Solid Edge part; units mm, degrees
sketch "Sketch1" plane through (0, 0, 0) normal (0, 0, 1) x (1, 0, 0)
  circle A0 centre (0, 41.891) radius 2.5
  line L0 (-5, 46.891) -> (5, 46.891)
  line L1 (5, 46.891) -> (5, 36.891)
  line L2 (5, 36.891) -> (-5, 36.891)
  line L3 (-5, 36.891) -> (-5, 46.891)
  circle A1 centre (0, -41.891) radius 2.5
  line L4 (-5, -46.891) -> (5, -46.891)
  line L5 (5, -46.891) -> (5, -36.891)
  line L6 (5, -36.891) -> (-5, -36.891)
  line L7 (-5, -36.891) -> (-5, -46.891)
  line L8 (-26, 36.891) -> (26, 36.891)
  line L9 (26, 36.891) -> (26, -36.891)
  line L10 (26, -36.891) -> (-26, -36.891)
  line L11 (-26, -36.891) -> (-26, 36.891)
  circle A2 centre (0, 15.851) radius 5
  dimension "D1" = 26
  dimension "D2" = 26
  dimension "D3" = 5
  dimension "D4" = 5
  dimension "D5" = 5
  dimension "D6" = 5
extrude "Protrusion1" add sketch "Sketch1" against normal blind 3
fillet "v_10" radius 10 4 edges at (26, -36.891, -1.5) (26, 36.891, -1.5) (-26, 36.891, -1.5) (-26, -36.891, -1.5)
fillet "v_5" radius 5 8 edges at (5, -46.891, -1.5) (-5, -46.891, -1.5) (5, -36.891, -1.5) (-5, -36.891, -1.5) (5, 46.891, -1.5) (5, 36.891, -1.5) (-5, 46.891, -1.5) (-5, 36.891, -1.5)
properties material "ABS Plastic, high impact"
The model under review builds one solid part; all positions refer to its coordinate system, in mm. A direction names the side the tool comes from. Give positions to 0.01 mm unless a question says otherwise; leave off trailing zeros. Write each loop counter-clockwise with the first axis right and the second up, starting at its lowest first coordinate (ties: lowest second). Pieces come first, ordered by that corner, then holes. Notation, with made-up numbers: M 29.25,-33.5 L 37.25,-33.5 A11 ccw 37.25,-17.5 Z; hole C 51,-17.5 d6. An arc over 180 degrees is marked long. Answer in a Markdown table with one row per item.
Item 1: Add section A-A on z = -0.8. State how many separate pieces and enclosed holes the cut face has, plus the area to 3 significant figures.
Check sheet entries:
| item | result |
|---|---|
| separate pieces | 1 |
| enclosed holes | 3 |
| area | 3,830 mm2 |
Item 2: Add section C-C on x = 7.5. Give the boundary of the cut face in (y, z), plus the area to 3 significant figures.
Check sheet entries:
| item | result |
|---|---|
| outline | M -37.56,-3 L 37.56,-3 L 37.56,0 L -37.56,0 Z |
| area | 225 mm2 |
Item 3: For line 1 along Y through (x, z) = (0, -2); line 2 along Y through (x, z) = (2, -1.1); line 3 along X through (y, z) = (18, -0.2), list the stretches that pass through material, from the lowest coordinate up.
Check sheet entries:
| item | result |
|---|---|
| line 1 | -46.89 to -44.39, -39.39 to 10.85, 20.85 to 39.39, 44.39 to 46.89 |
| line 2 | -46.47 to -43.39, -40.39 to 11.27, 20.43 to 40.39, 43.39 to 46.47 |
| line 3 | -26 to -4.51, 4.51 to 26 |
Item 4: Tool access review of faces 4 (the face through (0, 1, -3)), 5 (the face through (-13, -36.891, -1)), 6 (the face through (-13, 36.891, -1)), 7 (the face through (13, -36.891, -1)): name each direction out of +Z, -Z, +X, -X, +Y, -Y from which nothing blocks a thin tool from reaching the whole face with its end or side.
Check sheet entries:
| item | result |
|---|---|
| face 4 | -Z, +X, -X, +Y, -Y |
| face 5 | +Z, -Z, -X, -Y |
| face 6 | +Z, -Z, -X, +Y |
| face 7 | +Z, -Z, +X, -Y |
Item 5: Draft analysis for pull direction X (two halves, no side actions). For faces 1 (the face through (-0.54, -44.33, -1.48)), 2 (the face through (0, 1, 0)), 3 (the face through (3.497, 45.465, -1.521)), state which applies: +X half, -X half, draft (parallel to the pull), parting line (faces both ways), or undercut.
Check sheet entries:
| item | result |
|---|---|
| face 1 | undercut |
| face 2 | draft |
| face 3 | +X half |
Item 6: Add section B-B on x = -6. Give the boundary of the cut face in (y, z), plus the area to 3 significant figures.
Check sheet entries:
| item | result |
|---|---|
| outline | M -38.89,-3 L 38.89,-3 L 38.89,0 L -38.89,0 Z |
| area | 233 mm2 |
Item 7: For P1, Ø1.5, axis at x = -13, z = -1.5, coming from the -Y side; P2, Ø1.5, axis at x = -2.5, z = -2, coming from the +Y side, all flat-tipped, find the tip position at first contact; note any pin that passes through.
Check sheet entries:
| item | result |
|---|---|
| P1 | y = -36.89 |
| P2 | y = 46.57 |
